Verification items for the finished model (mm, model axes). Give positions to 0.01 mm unless a question says otherwise; leave off trailing zeros. Write each loop counter-clockwise with the first axis right and the second up, starting at its lowest first coordinate (ties: lowest second). Pieces come first, ordered by that corner, then holes. Notation, with made-up numbers: M 36,73.25 L 66,73.25 A14 ccw 66,77.25 Z; hole C 35,-1.75 d10. An arc over 180 degrees is marked long. Answer as a JSON object with one key per item and string values.
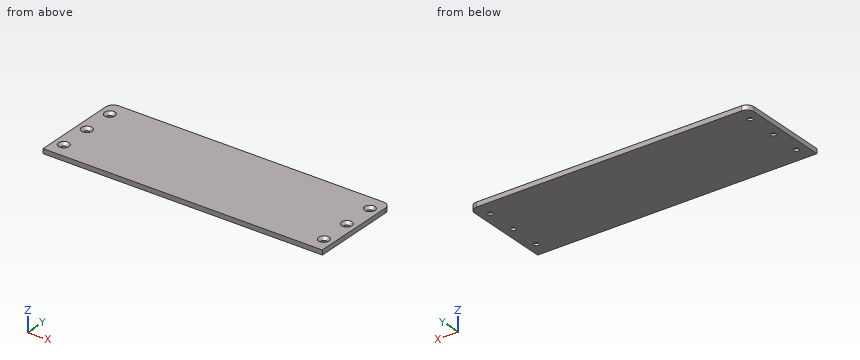
```python
from build123d import *

# Parameters (mm, degrees)
SKETCH1_W                                      = 180
SKETCH1_H                                      = 60
BOSS_EXTRUDE1_DEPTH                            = 3
FILLET1_R                                      = 5
CSK_FOR_M3_FLAT_HEAD_MACHINE_SCREW1_AT_2_COUNT = 2
CSK_FOR_M3_FLAT_HEAD_MACHINE_SCREW1_AT_2_PITCH = 20
CSK_FOR_M3_FLAT_HEAD_MACHINE_SCREW1_AT_3_COUNT = 2
CSK_FOR_M3_FLAT_HEAD_MACHINE_SCREW1_AT_3_PITCH = 40
CSK_FOR_M3_FLAT_HEAD_MACHINE_SCREW1_AT_4_COUNT = 2
CSK_FOR_M3_FLAT_HEAD_MACHINE_SCREW1_AT_4_PITCH = 167
CSK_FOR_M3_FLAT_HEAD_MACHINE_SCREW1_AT_5_COUNT = 2
CSK_FOR_M3_FLAT_HEAD_MACHINE_SCREW1_AT_5_PITCH = 168.193341129
CSK_FOR_M3_FLAT_HEAD_MACHINE_SCREW1_AT_6_COUNT = 2
CSK_FOR_M3_FLAT_HEAD_MACHINE_SCREW1_AT_6_PITCH = 171.723615149
CUT_EXTRUDE1_REACH                             = 96.916


with BuildPart() as part:
    # Sketch1 → Boss-Extrude1 (new body)
    with BuildSketch(Plane.XY):
        Rectangle(SKETCH1_W, SKETCH1_H)
    extrude(amount=BOSS_EXTRUDE1_DEPTH)

    # Fillet1
    fillet1_edges = [part.edges().sort_by_distance(p)[0] for p in [
        (-90, 30, 1.5),
        (90, 30, 1.5),
    ]]
    fillet(fillet1_edges, radius=FILLET1_R)

    # Sketch3 → CSK for M3 Flat Head Machine Screw1 (revolve, cut)
    with BuildSketch(Plane(origin=(-83.5, 20, 3), x_dir=(0, -1, 0), z_dir=(1, 0, 0))):
        Polygon((0, 0), (0, 3), (1.7, 3), (1.7, 1.7), (3.4, 0), align=None)
    csk_for_m3_flat_head_machine_screw1 = revolve(axis=Axis((-83.5, 20, 9.35), (0, 0, -1)), mode=Mode.SUBTRACT)

    # CSK for M3 Flat Head Machine Screw1 at 2: CSK for M3 Flat Head Machine Screw1 ×2
    with Locations(*[(0, -i * CSK_FOR_M3_FLAT_HEAD_MACHINE_SCREW1_AT_2_PITCH, 0) for i in range(1, CSK_FOR_M3_FLAT_HEAD_MACHINE_SCREW1_AT_2_COUNT)]):
        add(csk_for_m3_flat_head_machine_screw1, mode=Mode.SUBTRACT)

    # CSK for M3 Flat Head Machine Screw1 at 3: CSK for M3 Flat Head Machine Screw1 ×2
    with Locations(*[(0, -i * CSK_FOR_M3_FLAT_HEAD_MACHINE_SCREW1_AT_3_PITCH, 0) for i in range(1, CSK_FOR_M3_FLAT_HEAD_MACHINE_SCREW1_AT_3_COUNT)]):
        add(csk_for_m3_flat_head_machine_screw1, mode=Mode.SUBTRACT)

    # CSK for M3 Flat Head Machine Screw1 at 4: CSK for M3 Flat Head Machine Screw1 ×2
    with Locations(*[(i * CSK_FOR_M3_FLAT_HEAD_MACHINE_SCREW1_AT_4_PITCH, 0, 0) for i in range(1, CSK_FOR_M3_FLAT_HEAD_MACHINE_SCREW1_AT_4_COUNT)]):
        add(csk_for_m3_flat_head_machine_screw1, mode=Mode.SUBTRACT)

    # CSK for M3 Flat Head Machine Screw1 at 5: CSK for M3 Flat Head Machine Screw1 ×2
    with Locations(*[Vector(0.9929049442707555, -0.11891077176895277, 0) * (i * CSK_FOR_M3_FLAT_HEAD_MACHINE_SCREW1_AT_5_PITCH) for i in range(1, CSK_FOR_M3_FLAT_HEAD_MACHINE_SCREW1_AT_5_COUNT)]):
        add(csk_for_m3_flat_head_machine_screw1, mode=Mode.SUBTRACT)

    # CSK for M3 Flat Head Machine Screw1 at 6: CSK for M3 Flat Head Machine Screw1 ×2
    with Locations(*[Vector(0.9724929204096406, -0.2329324360262613, 0) * (i * CSK_FOR_M3_FLAT_HEAD_MACHINE_SCREW1_AT_6_PITCH) for i in range(1, CSK_FOR_M3_FLAT_HEAD_MACHINE_SCREW1_AT_6_COUNT)]):
        add(csk_for_m3_flat_head_machine_screw1, mode=Mode.SUBTRACT)

    # Sketch4 → Cut-Extrude1 (cut, up to next)
    with BuildSketch(Plane.XY.offset(3), mode=Mode.PRIVATE) as cut_extrude1_sk1:
        with BuildLine():
            Line((85, 30), (-85, 30))
            ThreePointArc((-85, 30), (-88.535533906, 28.535533906), (-90, 25))
            Line((-90, 25), (-90, -30))
            Line((-90, -30), (90, -30))
            Line((90, -30), (90, 25))
            ThreePointArc((90, 25), (88.535533906, 28.535533906), (85, 30))
        make_face()
        with BuildLine():
            Line((85, 29.7), (-85, 29.7))
            ThreePointArc((-85, 29.7), (-88.323401872, 28.323401872), (-89.7, 25))
            Line((-89.7, 25), (-89.7, -29.7))
            Line((-89.7, -29.7), (89.7, -29.7))
            Line((89.7, -29.7), (89.7, 25))
            ThreePointArc((89.7, 25), (88.323401872, 28.323401872), (85, 29.7))
        make_face(mode=Mode.SUBTRACT)
    cut_extrude1_tool1 = extrude(cut_extrude1_sk1.sketch, amount=-CUT_EXTRUDE1_REACH, mode=Mode.PRIVATE) & part.part
    add(cut_extrude1_tool1.solids().sort_by_distance((0, 29.810263, 3))[0], mode=Mode.SUBTRACT)


solid = part.part
```
1) Go/stop test with flat-tipped pins: pin 1 (5.5 mm diameter, centred on x = -83.5, y = 20, fed in from +Z); pin 2 (10 mm diameter, centred on x = 51, y = -2, fed in from -Z); pin 3 (2.5 mm diameter, centred on x = -83.5, y = 0, fed in from +Z); pin 4 (4 mm diameter, centred on x = 83.5, y = 0, fed in from +Z). Record where each tip stops, or that it passes through.
Completed:
{"pin 1": "stops at z = 2.35", "pin 2": "stops at z = 0", "pin 3": "passes through", "pin 4": "stops at z = 1.6"}
2) Section check A-A on y = 0. Record the boundary of the cut face in (x, z), and give its area (3 significant figures).
Completed:
{"outline": "M -89.7,0 L -85.2,0 L -85.2,1.3 L -86.9,3 L -89.7,3 Z; M -81.8,0 L 81.8,0 L 81.8,1.3 L 80.1,3 L -80.1,3 L -81.8,1.3 Z; M 85.2,0 L 89.7,0 L 89.7,3 L 86.9,3 L 85.2,1.3 Z", "area": "512 mm2"}
3) Thickness scan on L1, parallel to X at y = 0, z = 0.9; L2, parallel to Y at x = -83.5, z = 0.4; L3, parallel to X at y = 20.5, z = 0.35. Record the ranges inside material, lowest first.
Completed:
{"L1": "x = -89.7 to -85.2, -81.8 to 81.8, 85.2 to 89.7", "L2": "y = -29.7 to -21.7, -18.3 to -1.7, 1.7 to 18.3, 21.7 to 29.7", "L3": "x = -89.7 to -85.12, -81.88 to 81.88, 85.12 to 89.7"}
